Verification items for the finished model (mm, model axes). Round coordinates to 2 decimals unless told otherwise and drop trailing zeros. One line per item, written item: value. Start each with the question number.
Item 1: Draft check along Y on faces 1 (the face through (-57, -75, 1)), 2 (the face through (61, 1, 1)), 3 (the face through (-52.383, 70.33, 1.521)). Enter one of: +Y half, -Y half, draft (parallel to the pull), parting line (faces both ways), or undercut.
Item 2: Gauge pin test, flat ends, axial feed: pin 1 (1.6 mm diameter, centred on x = 39.16, y = -24.13, fed in from -Z); pin 2 (3 mm diameter, centred on x = -47.28, y = -47.28, fed in from -Z). Record the tip position at first contact, or that the pin passes through.
Item 3: Thickness scan on probe 1 along X at (y, z) = (71, 1.45); probe 2 along Y at (x, z) = (47.5, 1.15); probe 3 along Y at (x, z) = (-47, 1.6). Record the ranges inside material, lowest first. Write a range as from..to.
from build123d import *

# Parameters (mm, degrees)
PAD_DEPTH       = 3
SKETCH001_R     = 1.25
POCKET_DEPTH    = 3.001
SKETCH002_R     = 1.25
POCKET001_DEPTH = 3.001
SKETCH003_R     = 1
POCKET002_DEPTH = 3.001
SKETCH004_R     = 1.25
POCKET003_DEPTH = 3.001
SKETCH005_R     = 1.75
POCKET004_DEPTH = 3.001


with BuildPart() as part:
    # Sketch → Pad (new body)
    with BuildSketch(Plane.XY):
        Polygon((-61, 71), (-54, 78), (54, 78), (61, 71), (61, -71), (54, -78), (-54, -78), (-61, -71), align=None)
    extrude(amount=PAD_DEPTH)

    # Sketch001 (on Face10 of Pad) → Pocket (cut, through all)
    with BuildSketch(Plane.XY.offset(3)):
        with Locations((-42.5, 63)):
            Circle(SKETCH001_R)
        with Locations((42.5, 63)):
            Circle(SKETCH001_R)
        with Locations((-42.5, -63)):
            Circle(SKETCH001_R)
        with Locations((42.5, -63)):
            Circle(SKETCH001_R)
    extrude(amount=-POCKET_DEPTH, mode=Mode.SUBTRACT)

    # Sketch002 (on Face5 of Pocket) → Pocket001 (cut, through all)
    with BuildSketch(Plane.XY.offset(3)):
        with Locations((-38, 67.5)):
            Circle(SKETCH002_R)
        with Locations((38, 67.5)):
            Circle(SKETCH002_R)
        with Locations((38, -67.5)):
            Circle(SKETCH002_R)
        with Locations((-38, -67.5)):
            Circle(SKETCH002_R)
    extrude(amount=-POCKET001_DEPTH, mode=Mode.SUBTRACT)

    # Sketch003 (on Face5 of Pocket001) → Pocket002 (cut, through all)
    with BuildSketch(Plane.XY.offset(3)):
        with Locations((-42.12, 24.13)):
            Circle(SKETCH003_R)
        with Locations((-35.77, -24.13)):
            Circle(SKETCH003_R)
        with Locations((40.43, 24.13)):
            Circle(SKETCH003_R)
        with Locations((39.16, -24.13)):
            Circle(SKETCH003_R)
    extrude(amount=-POCKET002_DEPTH, mode=Mode.SUBTRACT)

    # Sketch004 (on Face5 of Pocket002) → Pocket003 (cut, through all)
    with BuildSketch(Plane.XY.offset(3)):
        with Locations((-47.28, 47.28)):
            Circle(SKETCH004_R)
        with Locations((47.28, 47.28)):
            Circle(SKETCH004_R)
        with Locations((-47.28, -47.28)):
            Circle(SKETCH004_R)
        with Locations((47.28, -47.28)):
            Circle(SKETCH004_R)
    extrude(amount=-POCKET003_DEPTH, mode=Mode.SUBTRACT)

    # Sketch005 (on Face5 of Pocket003) → Pocket004 (cut, through all)
    with BuildSketch(Plane.XY.offset(3)):
        with Locations((-54, 71)):
            Circle(SKETCH005_R)
        with Locations((54, 71)):
            Circle(SKETCH005_R)
        with Locations((-54, -71)):
            Circle(SKETCH005_R)
        with Locations((54, -71)):
            Circle(SKETCH005_R)
    extrude(amount=-POCKET004_DEPTH, mode=Mode.SUBTRACT)


solid = part.part
Response values:
1. face 1: -Y half
1. face 2: draft
1. face 3: undercut
2. pin 1: passes through
2. pin 2: stops at z = 0
3. probe 1: x = -61..-55.75, -52.25..52.25, 55.75..61
3. probe 2: y = -78..-48.51, -46.05..46.05, 48.51..78
3. probe 3: y = -78..-48.5, -46.06..46.06, 48.5..78
